Part print with two shaded views. Sizes in mm from the minimum x, y, z corner. Give positions to 0.01 mm unless a question says otherwise; leave off trailing zeros. Write each loop counter-clockwise with the first axis right and the second up, starting at its lowest first coordinate (ties: lowest second). Pieces come first, ordered by that corner, then holes. Notation, with made-up numbers: M 0.5,37.5 L 26.5,37.5 A22 cw 26.5,45.5 Z; hole C -25,-19.75 d1. An arc over 180 degrees is marked long. Return JSON: item names as keys, results as strings. Group by question number.
Q1. Band-saw the part on A-A, the plane z = 1.75. Give the cut face in (x, y), then the cut area to 3 significant figures.
Q2. Band-saw the part on C-C, the plane y = 3. Give the cut face in (x, z), then the cut area to 3 significant figures.
Q3. Band-saw the part on B-B, the plane x = 125. Give the cut face in (y, z).
Q4. Wall check: probe 1 along Y at (x, z) = (125, 3.4); probe 2 along Y at (x, z) = (123.5, 2.1); probe 3 along X at (y, z) = (10.25, 1.2). Give the ranges that are in metal, low to high.
Q5. Flat gauge pin, fed straight in: pin 1 Ø2.5 at (x, y) = (5, 3) entering from -Z. Where does the tip first touch, or does it go through?
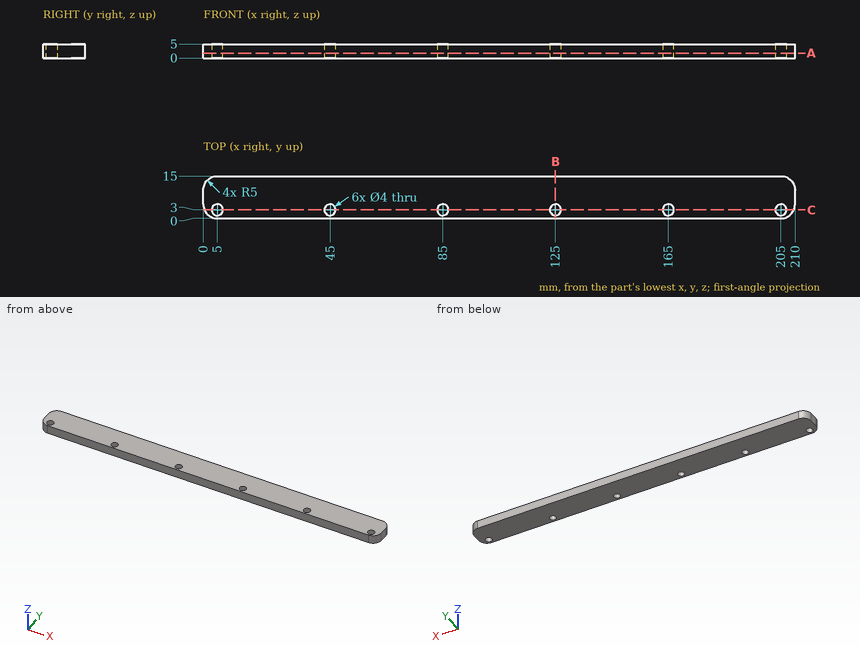
From the geometry:
{
 "1": {"outline": "M 0,5 A5 ccw 5,0 L 205,0 A5 ccw 210,5 L 210,10 A5 ccw 205,15 L 5,15 A5 ccw 0,10 Z; hole C 5,3 d4; hole C 45,3 d4; hole C 85,3 d4; hole C 125,3 d4; hole C 165,3 d4; hole C 205,3 d4", "area": "3,050 mm^2"},
 "2": {"outline": "M 0.42,0 L 3,0 L 3,5 L 0.42,5 Z; M 7,0 L 43,0 L 43,5 L 7,5 Z; M 47,0 L 83,0 L 83,5 L 47,5 Z; M 87,0 L 123,0 L 123,5 L 87,5 Z; M 127,0 L 163,0 L 163,5 L 127,5 Z; M 167,0 L 203,0 L 203,5 L 167,5 Z; M 207,0 L 209.58,0 L 209.58,5 L 207,5 Z", "area": "926 mm^2"},
 "3": {"outline": "M 0,0 L 1,0 L 1,5 L 0,5 Z; M 5,0 L 15,0 L 15,5 L 5,5 Z"},
 "4": {"probe 1": "y = 0 to 1, 5 to 15", "probe 2": "y = 0 to 1.68, 4.32 to 15", "probe 3": "x = 0.01 to 209.99"},
 "5": {"pin 1": "passes through"}
}
